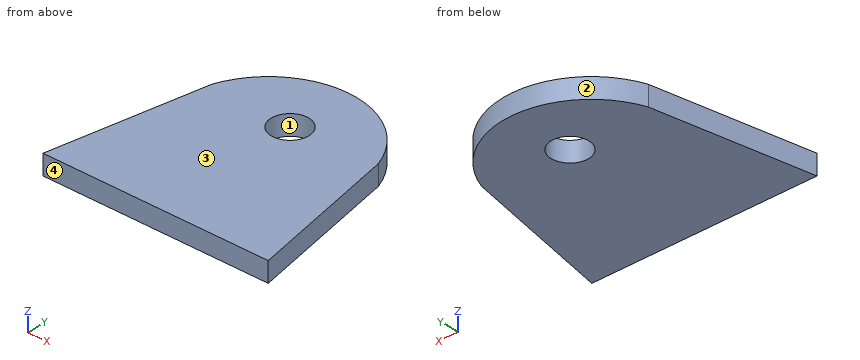
from build123d import *

# Parameters (mm, degrees)
SKETCH1_R           = 2.38125
BOSS_EXTRUDE1_DEPTH = 2.54


with BuildPart() as part:
    # Sketch1 → Boss-Extrude1 (new body)
    with BuildSketch(Plane.XY):
        with BuildLine():
            Line((0, 0), (28.575, 0))
            Line((28.575, 0), (24.855666251, 19.758430469))
            ThreePointArc((24.855666251, 19.758430469), (14.2875, 27.2161), (3.719333749, 19.758430469))
            Line((3.719333749, 19.758430469), (0, 0))
        make_face()
        with Locations((14.2875, 19.05)):
            Circle(SKETCH1_R, mode=Mode.SUBTRACT)
    extrude(amount=-BOSS_EXTRUDE1_DEPTH)


solid = part.part
Part model, mm, in its own coordinate system. Face numbers are marked on the shaded views. Give positions to 0.01 mm unless a question says otherwise; leave off trailing zeros. Write each loop counter-clockwise with the first axis right and the second up, starting at its lowest first coordinate (ties: lowest second). Pieces come first, ordered by that corner, then holes.
1) Pin check, flat tips, straight feed: pin 1 (1.5 mm diameter, centred on y = 19.5, z = -0.5, fed in from -X); pin 2 (1.5 mm diameter, centred on x = 4, z = -2, fed in from +Y). Stop position of each tip, or through.
Resolved:
pin 1: stops at x = 3.53
pin 2: stops at y = 21.9
2) Probe L1, parallel to Y at x = 12.5, z = -2.3; L2, parallel to X at y = 19.75, z = -2.25; L3, parallel to Y at x = 12.25, z = -1.8. List the from-to ranges inside material, lowest first.
Resolved:
L1: y = 0 to 17.48, 20.62 to 27.07
L2: x = 3.72 to 12.01, 16.56 to 24.86
L3: y = 0 to 17.82, 20.28 to 27.03
3) Cut at D-D on x = 26.75. Write the cut outline in (y, z).
Resolved:
outline: (0, -2.54) - (9.7, -2.54) - (9.7, 0) - (0, 0) - close
4) Two-plate mould, pull along Y, no slides. Class the marked faces 1, 2, 3 and 4: released by +Y, released by -Y, zero draft, split by the parting line, or undercut.
Resolved:
face 1: undercut
face 2: released by +Y
face 3: zero draft
face 4: released by -Y
5) Cut at C-C on x = 16.25. Write the cut outline in (y, z), then the cut area to 3 significant figures.
Resolved:
outline: (0, -2.54) - (17.7, -2.54) - (17.7, 0) - (0, 0) - close; (20.4, -2.54) - (27.04, -2.54) - (27.04, 0) - (20.4, 0) - close
area: 61.8 mm2
6) Cut at B-B on y = 19.05. Write the cut outline in (x, z), then the cut area to 3 significant figures.
Resolved:
outline: (3.59, -2.54) - (11.91, -2.54) - (11.91, 0) - (3.59, 0) - close; (16.67, -2.54) - (24.99, -2.54) - (24.99, 0) - (16.67, 0) - close
area: 42.3 mm2
